For this review, use the dimensioned drawing (mm, ordinates from the lowest corner) and the shaded views. Round coordinates to 2 decimals unless told otherwise and drop trailing zeros. Loops run counter-clockwise (first coordinate to the right, second up) from the corner with the lowest first, then second, coordinate; pieces in that order, holes last. Notation, with made-up numbers: (59, 58) -> (114, 58) arc R13 cw to (114, 65) -> close; hole circle Ø10 at (-39, 26). An arc over 180 degrees is marked (long way). Write each question's results on one line, items separated by ' | '. Start each with the question number.
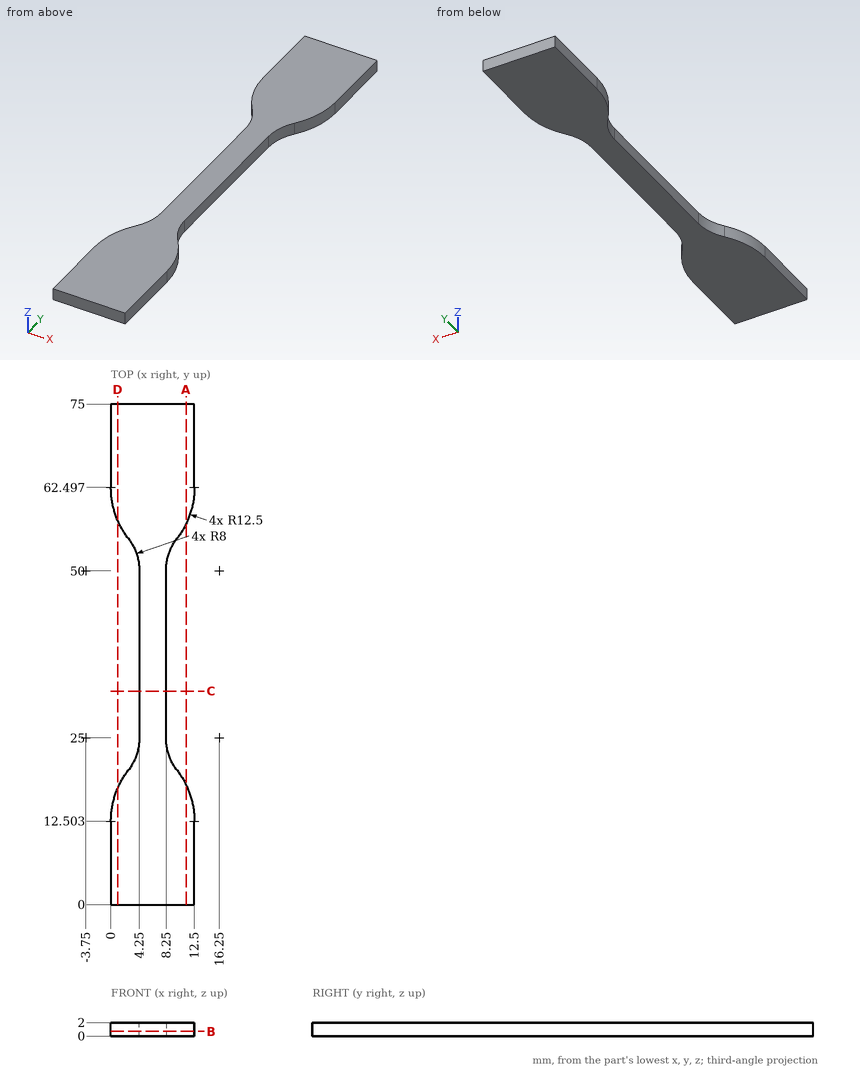
1) Take a section at D-D (x = 1). Write out the cut boundary in (y, z).
2) To check wall thickness, follow line 1 (Y direction, x = 3.25, z = 1.8) (1 decimal); line 2 (X direction, y = 41.5, z = 1.9); line 3 (Y direction, x = 1.5, z = 0.9) (1 decimal). State the ranges of each line that lie inside material, in increasing order. Write a range as from..to.
3) Take a section at B-B (z = 0.7). Write out the cut boundary in (x, y).
4) Insertion check: pin 1 (1 mm diameter, centred on y = 41.5, z = 1.5, fed in from -X). The pin has a flat end and moves straight along its axis. Give the tip position at first contact, or say it passes through.
5) Take a section at A-A (x = 11.25). Write out the cut boundary in (y, z).
6) Take a section at C-C (y = 32). Write out the cut boundary in (x, z).
Geometry check:
1) outline: (0, 0) -> (17.4, 0) -> (17.4, 2) -> (0, 2) -> close; (57.6, 0) -> (75, 0) -> (75, 2) -> (57.6, 2) -> close
2) line 1: y = 0..21.1, 53.9..75 | line 2: x = 4.25..8.25 | line 3: y = 0..18.4, 56.6..75
3) outline: (0, 0) -> (12.5, 0) -> (12.5, 12.5) arc R12.5 ccw to (9.91, 20.12) arc R8 cw to (8.25, 25) -> (8.25, 50) arc R8 cw to (9.91, 54.88) arc R12.5 ccw to (12.5, 62.5) -> (12.5, 75) -> (0, 75) -> (0, 62.5) arc R12.5 ccw to (2.59, 54.88) arc R8 cw to (4.25, 50) -> (4.25, 25) arc R8 cw to (2.59, 20.12) arc R12.5 ccw to (0, 12.5) -> close
4) pin 1: stops at x = 4.25
5) outline: (0, 0) -> (17.95, 0) -> (17.95, 2) -> (0, 2) -> close; (57.05, 0) -> (75, 0) -> (75, 2) -> (57.05, 2) -> close
6) outline: (4.25, 0) -> (8.25, 0) -> (8.25, 2) -> (4.25, 2) -> close
